The model under review builds one solid part; all positions refer to its coordinate system, in mm. A direction names the side the tool comes from. Give positions to 0.01 mm unless a question says otherwise; leave off trailing zeros. Order: outer loops, then holes, each group sorted by start corner. A loop starts at its lowest first (then second) coordinate and runs counter-clockwise, first axis right, second up. Notation, with made-up numbers: (-0.5, 74) - (28.5, 74) arc R30 ccw to (28.5, 108) - close; hole circle Ø2 at (60, 7). An arc over 180 degrees is marked (long way). Write item = value, one per line. Start each with the question number.
1. For P1, Ø9, axis at x = 0, y = -58, coming from the +Z side; P2, Ø1.5, axis at y = -40.5, z = 3.5, coming from the +X side; P3, Ø2, axis at x = -1.5, z = 1.5, coming from the +Y side; P4, Ø2.5, axis at y = -20.5, z = 2.5, coming from the -X side, all flat-tipped, find the tip position at first contact; note any pin that passes through.
2. Wall thickness on probe 1 along X at (y, z) = (-35, 0.3); probe 2 along Y at (x, z) = (1.75, 0.45); probe 3 along Y at (x, z) = (-1, 2.6): over which ranges is each line inside the solid? List them lowest first.
3. Machinability: for faces 1 (the flat face through (-8.5, -33, 2)), 2 (the flat face through (8.5, -32, 2)), 3 (the cylindrical face through (0.187, -66.498, 2.465)), which of the approach directions +Z, -Z, +X, -X, +Y, -Y give a long, thin tool a straight path to every point of the face, cutting with its end or side? Answer none if there is none.
4. We need section A-A, the plane x = 0. Give the boundary of the cut face in (y, z), and give its area (3 significant figures).
5. We need section D-D, the plane x = 3.5. Give the boundary of the cut face in (y, z), and give its area (3 significant figures).
6. We need section C-C, the plane y = 0. Give the boundary of the cut face in (x, z).
7. We need section B-B, the plane z = 2. Give the boundary of the cut face in (x, y), and give its area (3 significant figures).
8. Mouldability with a two-part tool opening along Y and no side actions: class faces 4 (the cylindrical face through (7.015, 2.675, 2.465)), 5 (the flat face through (0, -28, 5)), 6 (the cylindrical face through (8.658, -4.756, 2.535)) as pulls with the +Y half, pulls with the -Y half, needs draft (parallel to the pull), parting line crosses it, or undercut.
from build123d import *

# Parameters (mm, degrees)
SKETCH_1_R      = 1.5
SKETCH_1_R_2    = 2
SKETCH_1_R_3    = 5
EXTRUDE_1_DEPTH = 5
FILLET_1_R      = 15


with BuildPart() as part:
    # 草图1 → 凸台-拉伸1 (new body)
    with BuildSketch(Plane.XY):
        with BuildLine():
            Line((-8.5, -58), (-8.5, -4.242640687))
            ThreePointArc((-8.5, -4.242640687), (0, 9.5), (8.5, -4.242640687))
            Line((8.5, -4.242640687), (8.5, -58))
            ThreePointArc((8.5, -58), (0, -66.5), (-8.5, -58))
        make_face()
        with Locations((-5.629165125, 3.25)):
            Circle(SKETCH_1_R, mode=Mode.SUBTRACT)
        Circle(SKETCH_1_R_2, mode=Mode.SUBTRACT)
        with Locations((0, -58)):
            Circle(SKETCH_1_R_3, mode=Mode.SUBTRACT)
        with Locations((5.629165125, 3.25)):
            Circle(SKETCH_1_R, mode=Mode.SUBTRACT)
        with Locations((0, -6.5)):
            Circle(SKETCH_1_R, mode=Mode.SUBTRACT)
    extrude(amount=EXTRUDE_1_DEPTH)

    # 圆角1
    fillet_1_edges = [part.edges().sort_by_distance(p)[0] for p in [
        (-8.5, -4.242640687, 2.5),
        (8.5, -4.242640687, 2.5),
    ]]
    fillet(fillet_1_edges, radius=FILLET_1_R)


solid = part.part
Model answer:
q1.P1 = through
q1.P2 = 8.5
q1.P3 = 9.49
q1.P4 = -8.5
q2.probe_1 = -8.5 to 8.5
q2.probe_2 = -66.32 to -62.68, -53.32 to -0.97, 0.97 to 9.34
q2.probe_3 = -66.44 to -62.9, -53.1 to -7.62, -5.38 to -1.73, 1.73 to 9.45
q3.face_1 = +Z, -Z, -X, -Y
q3.face_2 = +Z, -Z, +X, -Y
q3.face_3 = +Z, -Z, -Y
q4.outline = (-66.5, 0) - (-63, 0) - (-63, 5) - (-66.5, 5) - close; (-53, 0) - (-8, 0) - (-8, 5) - (-53, 5) - close; (-5, 0) - (-2, 0) - (-2, 5) - (-5, 5) - close; (2, 0) - (9.5, 0) - (9.5, 5) - (2, 5) - close
q4.area = 295 mm2
q5.outline = (-65.75, 0) - (-61.57, 0) - (-61.57, 5) - (-65.75, 5) - close; (-54.43, 0) - (8.83, 0) - (8.83, 5) - (-54.43, 5) - close
q5.area = 337 mm2
q6.outline = (-9.5, 0) - (-2, 0) - (-2, 5) - (-9.5, 5) - close; (2, 0) - (9.5, 0) - (9.5, 5) - (2, 5) - close
q7.outline = (-9.11, -2.69) arc R15 cw to (-8.5, -6.93) - (-8.5, -58) arc R8.5 ccw to (8.5, -58) - (8.5, -6.93) arc R15 cw to (9.11, -2.69) arc R9.5 ccw (long way) to start; hole circle Ø3 at (-5.63, 3.25); hole circle Ø10 at (0, -58); hole circle Ø4 at (0, 0); hole circle Ø3 at (0, -6.5); hole circle Ø3 at (5.63, 3.25)
q7.area = 1,140 mm2
q8.face_4 = undercut
q8.face_5 = needs draft
q8.face_6 = pulls with the -Y half
